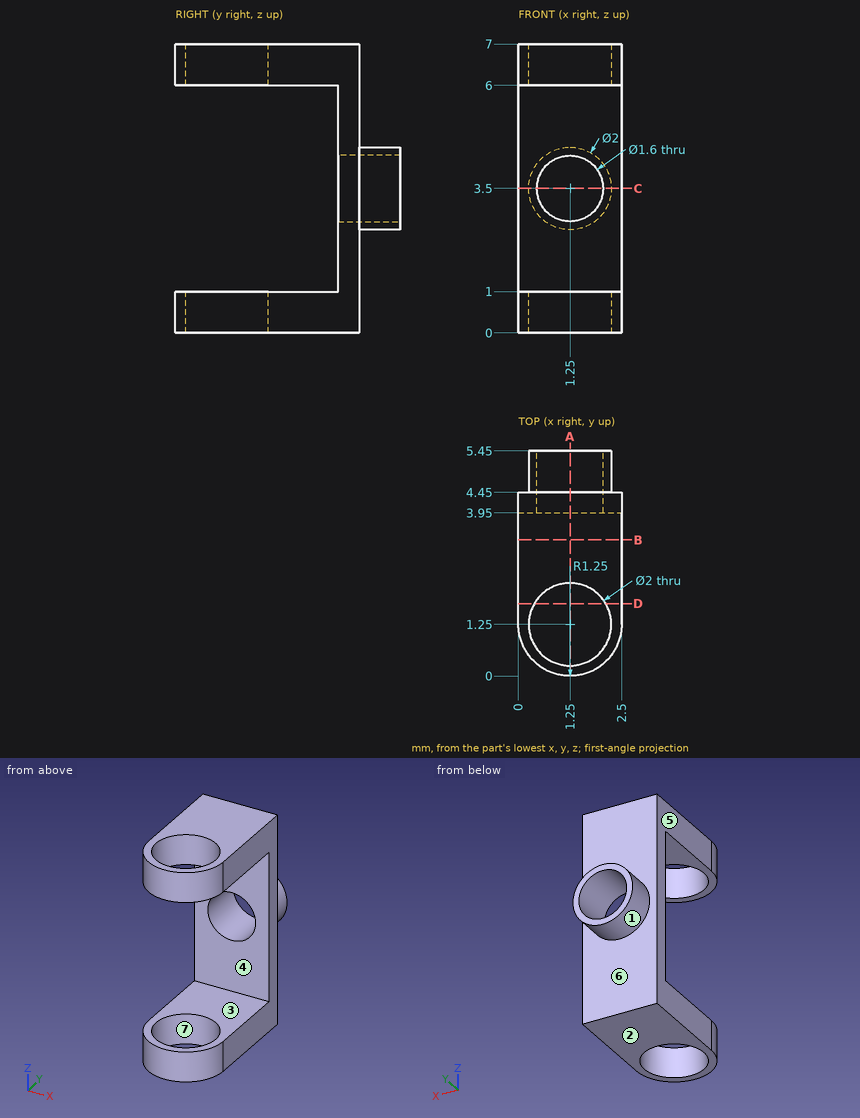
Source: three-view drawing plus pictorial views. Frame: mm from the lowest corner of the part. A direction names the side the tool comes from. Coordinates: 2 decimals unless noted, no trailing zeros. Order: outer loops, then holes, each group sorted by start corner. A loop starts at its lowest first (then second) coordinate and runs counter-clockwise, first axis right, second up.
1) Section D-D (y = 1.75). Return loops of the section in (x, z), then the cut area to 3 significant figures.
Result sheet:
outline: (0, 0) - (0.38, 0) - (0.38, 1) - (0, 1) - close; (0, 6) - (0.38, 6) - (0.38, 7) - (0, 7) - close; (2.12, 0) - (2.5, 0) - (2.5, 1) - (2.12, 1) - close; (2.12, 6) - (2.5, 6) - (2.5, 7) - (2.12, 7) - close
area: 1.54 mm2
2) Ray query, probe 1 along Y at (x, z) = (1.25, 6.55); probe 2 along Z at (x, y) = (0.8, 2.35); probe 3 along Y at (x, z) = (1.8, 6.5). Return the intervals inside material, ascending.
Result sheet:
probe 1: y = 0 to 0.25, 2.25 to 4.45
probe 2: z = 0 to 1, 6 to 7
probe 3: y = 0.13 to 0.41, 2.09 to 4.45
3) First-contact query: P1, Ø1, axis at x = 0.5, y = 2.5, coming from the -Z side; P2, Ø1.5, axis at x = 2, z = 6, coming from the +Y side. Flat tips, straight axial feed; report the tip coordinate or a pass-through.
Result sheet:
P1: stops at z = 0
P2: stops at y = 4.45
4) Section B-B (y = 3.3). Return loops of the section in (x, z), then the cut area to 3 significant figures.
Result sheet:
outline: (0, 0) - (2.5, 0) - (2.5, 1) - (0, 1) - close; (0, 6) - (2.5, 6) - (2.5, 7) - (0, 7) - close
area: 5.00 mm2
5) Section A-A (x = 1.25). Return loops of the section in (y, z).
Result sheet:
outline: (0, 0) - (0.25, 0) - (0.25, 1) - (0, 1) - close; (0, 6) - (0.25, 6) - (0.25, 7) - (0, 7) - close; (2.25, 0) - (4.45, 0) - (4.45, 2.5) - (5.45, 2.5) - (5.45, 2.7) - (3.95, 2.7) - (3.95, 1) - (2.25, 1) - close; (2.25, 6) - (3.95, 6) - (3.95, 4.3) - (5.45, 4.3) - (5.45, 4.5) - (4.45, 4.5) - (4.45, 7) - (2.25, 7) - close
6) Set-up query: the marked faces 1, 2 and 3. Return all of +Z, -Z, +X, -X, +Y, -Y with unobstructed straight access to the full face (end or side cutting, diameter ignored); none if empty.
Result sheet:
face 1: +Y
face 2: -Z, +X, -X, +Y, -Y
face 3: +X, -X, -Y
7) Draft query along Y for the marked faces 4, 5, 6 and 7. Return one class per face: released by +Y, released by -Y, zero draft, split by the parting line, or undercut.
Result sheet:
face 4: released by -Y
face 5: zero draft
face 6: released by +Y
face 7: undercut
8) Section C-C (z = 3.5). Return loops of the section in (x, y).
Result sheet:
outline: (0, 3.95) - (0.45, 3.95) - (0.45, 5.45) - (0.25, 5.45) - (0.25, 4.45) - (0, 4.45) - close; (2.05, 3.95) - (2.5, 3.95) - (2.5, 4.45) - (2.25, 4.45) - (2.25, 5.45) - (2.05, 5.45) - close
